Autodesk Inventor part; units mm, degrees
ref_plane "MSC_PF1" through (0, 0, 0) normal (1, 0, 0) x (0, 1, 0)
ref_plane "MSC_PT1" through (0, 0, 0) normal (0, 0, -1) x (-1, 0, 0)
ref_plane "YZ Plane" through (0, 0, 0) normal (1, 0, 0) x (0, 1, 0)
sketch "Sketch1" plane through (0, 0, 0) normal (0, 1, 0) x (-1, 0, 0)
  point P0 (0, 0)
sketch "Sketch2" plane through (0, 0, 0) normal (0, 1, 0) x (-1, 0, 0)
  line L0 (-2, -20) -> (0, -20)
  line L1 (-2, -2.3) -> (-2, -20)
  line L2 (-4, -0.3) -> (-2, -2.3)
  line L3 (-4, 0) -> (-4, -0.3)
  line L4 (0, 0) -> (-4, 0)
  line L5 (0, -20) -> (0, 0)
  line L6 (0, -20) -> (0, 0)
  line L7 (0, -24) -> (0, 4)
  line L8 (0.8, 0) -> (-4.8, 0)
  dimension "d3" = 4
  dimension "d5" = 2
  dimension "d7" = 20
  dimension "ParC" = 0.3
  dimension "d22" = 0
  dimension "d23" = 0
  dimension "d43" = 45
revolve "Revolution1" add sketch "Sketch2" angle 360 about axis through (0, 0, -20) along (0, 0, -1)
sketch "Sketch3" plane through (0, 0, 0) normal (0, 0, 1) x (1, 0, 0)
  line L0 (-1.25, 0.7217) -> (-1.25, -0.7217)
  line L1 (0, 1.4434) -> (-1.25, 0.7217)
  line L2 (1.25, 0.7217) -> (0, 1.4434)
  line L3 (1.25, -0.7217) -> (1.25, 0.7217)
  line L4 (0, -1.4434) -> (1.25, -0.7217)
  line L5 (-1.25, -0.7217) -> (0, -1.4434)
  circle A0 centre (0, 0) radius 1.25 construction
  circle A1 centre (0, 0) radius 2 construction
  dimension "d11" = 2.5
  dimension "d13" = 120
  dimension "d15" = 120
extrude "Extrusion1" cut sketch "Sketch3" against normal blind 1.8
fillet "Fillet1" radius 0.2 1 edges at (-2, 0, -2.3)
chamfer "Chamfer1" distance 0.35 angle 45 1 edges at (-2, 0, -20) measured on face at (-0.9288, -1.7713, -14.1276)
thread "Thread1"
ref_plane "MSC_PF1" through (0, 0, 0) normal (1, 0, 0) x (0, 1, 0)
ref_plane "MSC_PT1" through (0, 0, 0) normal (0, 0, -1) x (-1, 0, 0)
equation "\"d3\" = 0.5 * dk"
equation "\"d5\" = 0.5 * NND"
equation "\"d7\" = NLG"
equation "\"d43\" = 0.5 * ang"
equation "\"d18\" = r"
equation "\"d19\" = 0.5 * PTC"
equation "\"d39\" = 0.5 * PTC"
equation "\"d11\" = ParS"
equation "\"d16\" = ParT"
equation "\"NND\" = 4"
equation "\"PTC\" = 0.7"
equation "\"dk\" = 8"
equation "\"ParK\" = 2.3"
equation "\"ParS\" = 2.5"
equation "\"ParT\" = 1.8"
equation "\"r\" = 0.2"
equation "\"NLG\" = 20"
equation "\"ang\" = 90deg"
equation "\"THREADDIA\" = NND"
properties part number "ISO 10642 - M4x20" material "Steel, Mild"
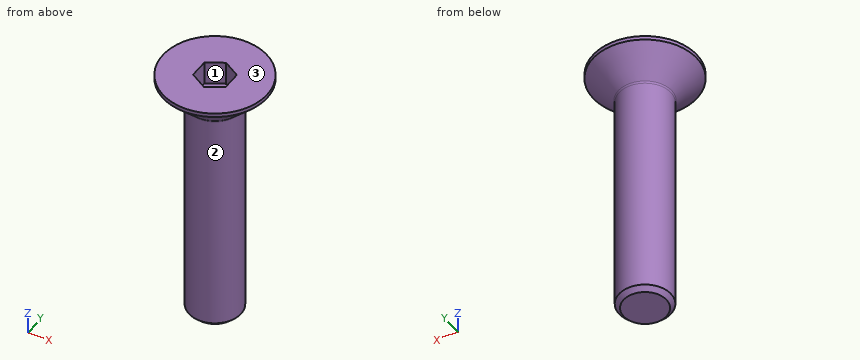
For this review, take the finished solid that the model builds, in its own axes (mm). Face numbers are marked on the shaded views. Round coordinates to 2 decimals unless told otherwise and drop trailing zeros. Write each loop counter-clockwise with the first axis right and the second up, starting at its lowest first coordinate (ties: lowest second). Pieces come first, ordered by that corner, then holes. Notation, with made-up numbers: (75, 60.5) - (89, 60.5) arc R17 cw to (89, 89.5) - close; hole circle Ø3 at (-27, -10). An arc over 180 degrees is marked (long way). Answer as a JSON object with one key per item and string values.
1. We need section A-A on z = -12.5. Give the boundary of the cut face in (x, y).
Response values:
{"outline": "circle Ø4 at (0, 0)"}
2. To check wall thickness, follow line 1 along Z through (x, y) = (2.75, 1.75); line 2 along Z through (x, y) = (-0.25, 2.75); line 3 along X through (y, z) = (0, -10). State the ranges of each line that lie inside material, in increasing order.
Response values:
{"line 1": "z = -1.04 to 0", "line 2": "z = -1.54 to 0", "line 3": "x = -2 to 2"}
3. Draft analysis for pull direction Y (two halves, no side actions). For the marked faces 1, 2 and 3, state which applies: +Y half, -Y half, draft (parallel to the pull), parting line (faces both ways), or undercut.
Response values:
{"face 1": "undercut", "face 2": "parting line", "face 3": "draft"}
4. For pin 1 Ø1.5 at (y, z) = (-1.5, -13.5) entering from -X; pin 2 Ø2 at (x, z) = (0.5, -13.5) entering from +Y; pin 3 Ø1.5 at (x, z) = (0.5, -14.5) entering from -Y, all flat-tipped, find the tip position at first contact; note any pin that passes through.
Response values:
{"pin 1": "stops at x = -1.85", "pin 2": "stops at y = 2", "pin 3": "stops at y = -2"}
